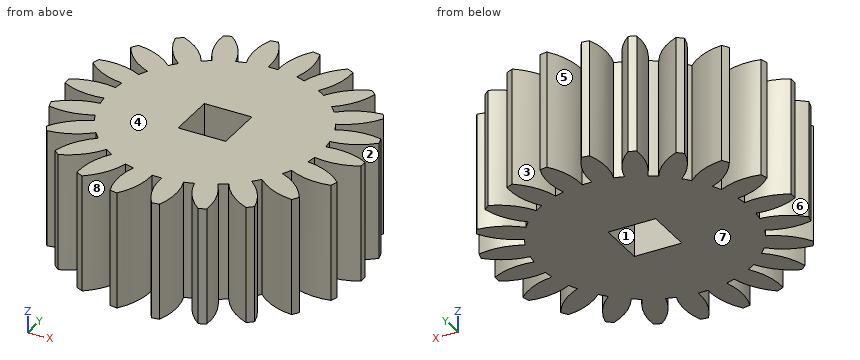
Autodesk Inventor part; units mm, degrees
ref_plane "YZ Plane" through (0, 0, 0) normal (1, 0, 0) x (0, 1, 0)
ref_plane "XZ Plane" through (0, 0, 0) normal (0, 1, 0) x (-1, 0, 0)
ref_plane "XY Plane" through (0, 0, 0) normal (0, 0, 1) x (1, 0, 0)
sketch "Sketch1" plane through (0, 0, 0) normal (0, 0, 1) x (1, 0, 0)
  circle A0 centre (0, 0) radius 12.5
  circle A1 centre (0, 0) radius 9
  line L0 (-12.5, 0) -> (12.5, 0)
  line L1 (-2.025, -2.025) -> (2.025, -2.025)
  line L2 (2.025, -2.025) -> (2.025, 2.025)
  line L3 (2.025, 2.025) -> (-2.025, 2.025)
  line L4 (-2.025, 2.025) -> (-2.025, -2.025)
  line L5 (-2.025, -2.025) -> (2.025, 2.025) construction
  line L6 (2.025, -2.025) -> (-2.025, 2.025) construction
  dimension "d0" = 25
  dimension "d1" = 18
  dimension "d7" = 4.05
extrude "Extrusion1" add sketch "Sketch1" along normal blind 10 contours L0 L2 L3 L4 A1 | A1 L0 L4 L1 L2
sketch "Sketch2" plane through (0, 0, 10) normal (0, 0, 1) x (1, 0, 0)
  line L0 (0, 0) -> (9, 0)
  circle A0 centre (0, 0) radius 9
  circle A1 centre (0, 0) radius 12.6
  arc A2 (12.5958, 0.325) -> (8.9574, 0.875) centre (10.0019, -4.5249) ccw
  arc A3 (8.9574, -0.875) -> (12.5958, -0.325) centre (10.0019, 4.5249) ccw
  point P0 (8.9574, -0.875)
  point P1 (12.5958, -0.325)
  dimension "d17" = 25.2
  dimension "d26" = 0.65
  dimension "d27" = 1.75
  dimension "d28" = 5.5
extrude "Extrusion2" add sketch "Sketch2" against normal blind 10 contours A0 A2 A1 A3 picked at (10.613, 0.2616)
pattern_circular "Circular Pattern1" count 22 over 360 about axis through (0, 0, -10) along (0, 0, 1) of "Extrusion2"
properties part number "Pinion Gear FV"
Source: CAD feature listing. Evaluate the final solid. Frame: model axes, mm. Face numbers are marked on the shaded views. A direction names the side the tool comes from. Coordinates: 2 decimals unless noted, no trailing zeros. Loops run counter-clockwise (first coordinate to the right, second up) from the corner with the lowest first, then second, coordinate; pieces in that order, holes last. Notation, with made-up numbers: (57.25, 85.5) - (101.25, 85.5) arc R15 cw to (101.25, 101.5) - close; hole circle Ø10 at (71.25, 60.5). An arc over 180 degrees is marked (long way). One line per item, written item: value. Start each with the question number.
1. Section A-A (x = -6). Return the cut outline in (y, z), and give its area (3 significant figures).
2. Mould query, pull axis X, two halves, no side actions, for the marked faces 5, 6, 7 and 8. Classes: pulls with the +X half, pulls with the -X half, needs draft (parallel to the pull), parting line crosses it, or undercut.
3. Contact query for flat-ended pins moving along their axis: P1, Ø3, axis at x = 8, z = 2, coming from the -Y side; P2, Ø2, axis at x = 4, z = 4, coming from the -Y side; P3, Ø4, axis at x = 5.5, z = 3.5, coming from the +Y side. Output: stop coordinate, or through.
4. Ray query, L1, parallel to X at y = 10, z = 5.5; L2, parallel to Y at x = -7.5, z = 6.5; L3, parallel to Y at x = -1.5, z = 5.25 (3 decimals). Return the intervals inside material, ascending.
5. Set-up query: the marked faces 1, 2, 3 and 4. Return all of +Z, -Z, +X, -X, +Y, -Y with unobstructed straight access to the full face (end or side cutting, diameter ignored); none if empty.
Verdict:
1. outline: (-8.4, 0) - (8.4, 0) - (8.4, 10) - (-8.4, 10) - close
1. area: 168 mm2
2. face 5: undercut
2. face 6: pulls with the -X half
2. face 7: needs draft
2. face 8: undercut
3. P1: stops at y = -9.73
3. P2: stops at y = -11.59
3. P3: stops at y = 11.59
4. L1: x = -5.45 to -3.53, -2.42 to -0.45, 0.45 to 2.42, 3.53 to 5.45
4. L2: y = -9.51 to -7.18, -5.95 to 5.95, 7.18 to 9.51
4. L3: y = -12.51 to -2.025, 2.025 to 12.51
5. face 1: +Z, -Z
5. face 2: +Z, -Z, +X
5. face 3: +Z, -Z, +Y
5. face 4: +Z, +X, -X, +Y, -Y
